from build123d import *

# Parameters (mm, degrees)
SKETCH3_R           = 12.5
BOSS_EXTRUDE1_DEPTH = 110
SKETCH4_R           = 12.5
BOSS_EXTRUDE2_DEPTH = 18.5
CHAMFER1_SIZE       = 2
SKETCH5_R           = 8
CUT_EXTRUDE1_DEPTH  = 18.5


with BuildPart() as part:
    # Sketch3 → Boss-Extrude1 (new body)
    with BuildSketch(Plane.XY):
        Circle(SKETCH3_R)
    extrude(amount=BOSS_EXTRUDE1_DEPTH)

    # Sketch4 → Boss-Extrude2 (add)
    with BuildSketch(Plane(origin=(0, 0, 0), x_dir=(0, 0, -1), z_dir=(1, 0, 0))):
        with Locations((-55, 0)):
            Circle(SKETCH4_R)
    extrude(amount=BOSS_EXTRUDE2_DEPTH)

    # Chamfer1
    chamfer1_edges = [part.edges().sort_by_distance(p)[0] for p in [
        (-12.5, 0, 0),
        (-12.5, 0, 110),
    ]]
    chamfer(chamfer1_edges, length=CHAMFER1_SIZE)

    # Sketch5 → Cut-Extrude1 (cut)
    with BuildSketch(Plane(origin=(18.5, 0, 0), x_dir=(0, 0, -1), z_dir=(1, 0, 0))):
        with Locations((-55, 0)):
            Circle(SKETCH5_R)
    extrude(amount=-CUT_EXTRUDE1_DEPTH, mode=Mode.SUBTRACT)


solid = part.part
The listing builds one solid part. Answer for the finished solid, in the listing's coordinates (mm). A direction names the side the tool comes from. Coordinates: 2 decimals unless noted, no trailing zeros. Order: outer loops, then holes, each group sorted by start corner. A loop starts at its lowest first (then second) coordinate and runs counter-clockwise, first axis right, second up. Notation, with made-up numbers: (-25, 15.25) -> (2, 15.25) arc R27 ccw to (2, 32.25) -> close; hole circle Ø2 at (-27, 16.5). An arc over 180 degrees is marked (long way). Answer in a Markdown table with one row per item. Add a question column.
Item 1: Each of these flat-tipped pins is pushed along its axis until it touches: P1, Ø4, axis at y = -8.5, z = 37.5, coming from the +X side; P2, Ø8, axis at y = -3.5, z = 83, coming from the -X side; P3, Ø6, axis at y = 8, z = 63, coming from the -X side; P4, Ø3, axis at y = 4, z = 62, coming from the -X side. Where does it stop, or does it pass through?
Item 2: Which of the six approach directions +Z, -Z, +X, -X, +Y, -Y give full straight-line access (tool end or side, diameter ignored) to faces 4 (the face through (18.5, 0.2, 46.8)), 5 (the face through (0, 0, 55)), 6 (the face through (-12.488, 0.55, 54.258))?
Item 3: Determine the mould class of faces 1 (the face through (0, 0, 110)), 2 (the face through (9.38, -4.868, 61.349)), 3 (the face through (0, 0, 0)) for opening direction Z: +Z half, -Z half, draft (parallel to the pull), parting line (faces both ways), or undercut.
Item 4: Find section C-C (z = 27.5). Write down the section's boundary in (x, y).
Item 5: Find the intervals of material crossed by L1, parallel to Y at x = 7.5, z = 55; L2, parallel to Z at x = 13, y = 3; L3, parallel to X at y = -0.5, z = 28, in increasing order. Write a range as from..to.
Item 6: Find section A-A (y = 0). Write down the section's boundary in (x, z), then the cut area to 3 significant figures.
Item 7: Find section B-B (z = 55). Write down the section's boundary in (x, y).
Result set:
| question | item | result |
|---|---|---|
| 1 | P1 | stops at x = 10.68 |
| 1 | P2 | stops at x = -12.5 |
| 1 | P3 | stops at x = -11.46 |
| 1 | P4 | stops at x = -12.25 |
| 2 | face 4 | +Z, -Z, +X, +Y, -Y |
| 2 | face 5 | +X |
| 2 | face 6 | none |
| 3 | face 1 | +Z half |
| 3 | face 2 | undercut |
| 3 | face 3 | -Z half |
| 4 | outline | circle Ø25 at (0, 0) |
| 5 | L1 | y = -12.5..-8, 8..12.5 |
| 5 | L2 | z = 42.87..47.58, 62.42..67.13 |
| 5 | L3 | x = -12.49..12.49 |
| 6 | outline | (-12.5, 2) -> (-10.5, 0) -> (10.5, 0) -> (12.5, 2) -> (12.5, 42.5) -> (18.5, 42.5) -> (18.5, 47) -> (0, 47) -> (0, 63) -> (18.5, 63) -> (18.5, 67.5) -> (12.5, 67.5) -> (12.5, 108) -> (10.5, 110) -> (-10.5, 110) -> (-12.5, 108) -> close |
| 6 | area | 2,600 mm² |
| 7 | outline | (0, -12.5) -> (18.5, -12.5) -> (18.5, -8) -> (0, -8) -> (0, 8) -> (18.5, 8) -> (18.5, 12.5) -> (0, 12.5) arc R12.5 ccw to start |
